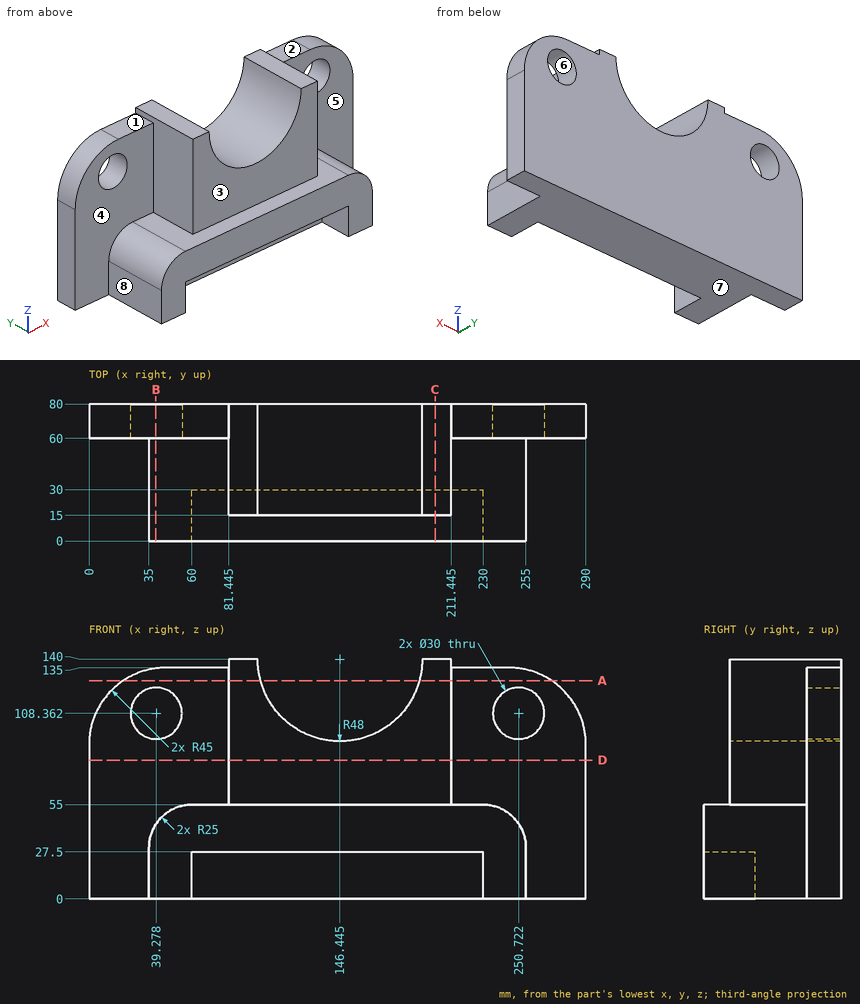
Input: dimensioned drawing with shaded views. Units: mm. Origin: part minimum x, y, z. A direction names the side the tool comes from. Give positions to 0.01 mm unless a question says otherwise; leave off trailing zeros. Loops run counter-clockwise (first coordinate to the right, second up) from the corner with the lowest first, then second, coordinate; pieces in that order, holes last. Notation, with made-up numbers: (-19.5, 12) -> (14.5, 12) arc R21 ccw to (14.5, 43) -> close; hole circle Ø9 at (43, 66.5). An arc over 180 degrees is marked (long way). Use a Markdown table: item, result. Add a question column.
1) Section query B-B, the plane x = 39. Return the cut outline in (y, z) (1 decimal).
2) Section query C-C, the plane x = 202. Return the cut outline in (y, z).
3) Section query A-A, the plane z = 127.5. Return the cut outline in (x, y) (1 decimal), then the cut area to 3 significant figures.
4) Line query: line 1 along X through (y, z) = (16, 12.5); line 2 along Y through (x, z) = (113, 20.5); line 3 along Y through (x, z) = (107, 107.5). Output: solid intervals per line, ascending. Write a range as [from, to].
5) Pull-direction query (X, two-part tool) for the marked faces 6, 7 and 8; classes: +X half, -X half, draft (parallel to the pull), parting line (faces both ways), or undercut.
6) Section query D-D, the plane z = 81. Return the cut outline in (x, y) (1 decimal).
7) First-contact query: pin 1 (3 mm diameter, centred on y = 11, z = 50.5, fed in from +X); pin 2 (5 mm diameter, centred on y = 46, z = 31, fed in from -X); pin 3 (12 mm diameter, centred on x = 145.5, z = 90, fed in from -Y); pin 4 (4 mm diameter, centred on x = 140.5, y = 30.5, fed in from -Z). Flat tips, straight axial feed; report the tip coordinate or a pass-through.
8) Reachability of the marked faces 1, 2, 3, 4 and 5 from +Z, -Z, +X, -X, +Y, -Y: full face, straight path, thin tool, end or side. Return the list, or none.
Numbers:
| question | item | result |
|---|---|---|
| 1 | outline | (0, 0) -> (80, 0) -> (80, 93.4) -> (60, 93.4) -> (60, 43.6) -> (0, 43.6) -> close; (60, 123.4) -> (80, 123.4) -> (80, 134.6) -> (60, 134.6) -> close |
| 2 | outline | (0, 27.5) -> (30, 27.5) -> (30, 0) -> (80, 0) -> (80, 140) -> (15, 140) -> (15, 55) -> (0, 55) -> close |
| 3 | outline | (20.1, 60) -> (81.4, 60) -> (81.4, 15) -> (100.1, 15) -> (100.1, 80) -> (20.1, 80) -> close; (192.8, 15) -> (211.4, 15) -> (211.4, 60) -> (269.9, 60) -> (269.9, 80) -> (192.8, 80) -> close |
| 3 | area | 4,820 mm2 |
| 4 | line 1 | x = [35, 60], [230, 255] |
| 4 | line 2 | y = [30, 80] |
| 4 | line 3 | y = [15, 80] |
| 5 | face 6 | undercut |
| 5 | face 7 | draft |
| 5 | face 8 | -X half |
| 6 | outline | (0, 60) -> (81.4, 60) -> (81.4, 15) -> (211.4, 15) -> (211.4, 60) -> (290, 60) -> (290, 80) -> (0, 80) -> close |
| 7 | pin 1 | stops at x = 246.25 |
| 7 | pin 2 | stops at x = 35 |
| 7 | pin 3 | stops at y = 15 |
| 7 | pin 4 | stops at z = 0 |
| 8 | face 1 | +Z, -X, +Y, -Y |
| 8 | face 2 | +Z, +X, +Y, -Y |
| 8 | face 3 | +Z, +X, -X, -Y |
| 8 | face 4 | +Z, -X, -Y |
| 8 | face 5 | +Z, +X, -Y |
